CAD build for the part. Positions are in the model's coordinates, mm. A direction names the side the tool comes from. Give positions to 0.01 mm unless a question says otherwise; leave off trailing zeros. Loops run counter-clockwise (first coordinate to the right, second up) from the corner with the lowest first, then second, coordinate; pieces in that order, holes last.
Item 1: Saw through at A-A on x = -11. Give the cut face in (y, z), plus the area to 3 significant figures.
Item 2: Mould opens along X. For faces 1 (the flat face through (-11.5, 2, 0)), 2 (the flat face through (18.75, 2, 0)), 3 (the cylindrical face through (-17.32, 2.54, 7.5)), 4 (the flat face through (0, 0, 8)) say: released by +X, released by -X, zero draft, split by the parting line, or undercut.
Item 3: Saw through at B-B on y = 3.75. Give the cut face in (x, z).
Item 4: Saw through at D-D on z = 0.75. Give the cut face in (x, y).
Item 5: Probe probe 1 along X at (y, z) = (1.4, 0); probe 2 along Z at (x, y) = (2, 0.55); probe 3 along X at (y, z) = (2.9, -3). List the from-to ranges inside material, lowest first.
Item 6: Drop flat-ended pins along their axis: P1, Ø1, axis at y = 3, z = -6, coming from the -X side; P2, Ø3.5, axis at x = 14.1, z = 0, coming from the +Y side; P3, Ø3, axis at y = 1, z = -6.5, coming from the +X side. Give the stop position or say it passes through.
Item 7: Saw through at C-C on z = 4.5. Give the cut face in (x, y).
Item 8: Which spindle directions (+Z, -Z, +X, -X, +Y, -Y) get a long thin tool onto all of the face, cutting with end or side? Do faces 5 (the cylindrical face through (-16.85, 3.77, -0.06)), 6 (the flat face through (0, 2, 7.1)), 7 (the cylindrical face through (17.25, 2.54, 7.57)). Say none if no direction does.
from build123d import *

# Parameters (mm, degrees)
SKETCH1_W           = 37.5
SKETCH1_H           = 18
SKETCH1_R           = 1.55
SKETCH1_W_2         = 23
SKETCH1_H_2         = 14.2
BOSS_EXTRUDE1_DEPTH = 5
SKETCH2_R           = 1.55
CUT_EXTRUDE1_DEPTH  = 2.5
FILLET1_R           = 5


with BuildPart() as part:
    # Sketch1 → Boss-Extrude1 (new body)
    with BuildSketch(Plane(origin=(0, 0, 0), x_dir=(1, 0, 0), z_dir=(0, 1, 0))):
        Rectangle(SKETCH1_W, SKETCH1_H)
        with Locations((-14.1, 0)):
            Circle(SKETCH1_R, mode=Mode.SUBTRACT)
        with Locations((14.1, 0)):
            Circle(SKETCH1_R, mode=Mode.SUBTRACT)
        Rectangle(SKETCH1_W_2, SKETCH1_H_2, mode=Mode.SUBTRACT)
    extrude(amount=BOSS_EXTRUDE1_DEPTH)

    # Sketch2 → Cut-Extrude1 (cut)
    with BuildSketch(Plane(origin=(0, 5, 0), x_dir=(1, 0, 0), z_dir=(0, 1, 0))):
        with BuildLine():
            ThreePointArc((11.5, 0.895823643), (12.503286973, 2.238974656), (14.1, 2.75))
            Line((14.1, 2.75), (11.5, 2.75))
            Line((11.5, 2.75), (11.5, 0.895823643))
        make_face()
        with BuildLine():
            Line((11.5, -2.75), (14.1, -2.75))
            ThreePointArc((14.1, -2.75), (12.503286973, -2.238974656), (11.5, -0.895823643))
            Line((11.5, -0.895823643), (11.5, -2.75))
        make_face()
        with BuildLine():
            ThreePointArc((16.85, 0), (16.044543648, 1.944543648), (14.1, 2.75))
            ThreePointArc((14.1, 2.75), (12.503286973, 2.238974656), (11.5, 0.895823643))
            Line((11.5, 0.895823643), (11.5, -0.895823643))
            ThreePointArc((11.5, -0.895823643), (12.503286973, -2.238974656), (14.1, -2.75))
            ThreePointArc((14.1, -2.75), (16.044543648, -1.944543648), (16.85, 0))
        make_face()
        with Locations((14.1, 0)):
            Circle(SKETCH2_R, mode=Mode.SUBTRACT)
        with BuildLine():
            ThreePointArc((-11.5, -0.895823643), (-12.503286973, -2.238974656), (-14.1, -2.75))
            Line((-14.1, -2.75), (-11.5, -2.75))
            Line((-11.5, -2.75), (-11.5, -0.895823643))
        make_face()
        with BuildLine():
            Line((-11.5, 2.75), (-14.1, 2.75))
            ThreePointArc((-14.1, 2.75), (-12.503286973, 2.238974656), (-11.5, 0.895823643))
            Line((-11.5, 0.895823643), (-11.5, 2.75))
        make_face()
        with BuildLine():
            ThreePointArc((-11.5, 0.895823643), (-12.503286973, 2.238974656), (-14.1, 2.75))
            ThreePointArc((-14.1, 2.75), (-16.85, 0), (-14.1, -2.75))
            ThreePointArc((-14.1, -2.75), (-12.503286973, -2.238974656), (-11.5, -0.895823643))
            Line((-11.5, -0.895823643), (-11.5, 0.895823643))
        make_face()
        with Locations((-14.1, 0)):
            Circle(SKETCH2_R, mode=Mode.SUBTRACT)
    extrude(amount=-CUT_EXTRUDE1_DEPTH, mode=Mode.SUBTRACT)

    # Fillet1
    fillet1_edges = [part.edges().sort_by_distance(p)[0] for p in [
        (18.75, 2.5, 9),
        (-18.75, 2.5, 9),
        (-18.75, 2.5, -9),
        (18.75, 2.5, -9),
    ]]
    fillet(fillet1_edges, radius=FILLET1_R)


solid = part.part
Results below:
1. outline: (0, -9) - (5, -9) - (5, -7.1) - (0, -7.1) - close; (0, 7.1) - (5, 7.1) - (5, 9) - (0, 9) - close
1. area: 19.0 mm2
2. face 1: undercut
2. face 2: released by +X
2. face 3: released by -X
2. face 4: zero draft
3. outline: (-18.75, -4) arc R5 ccw to (-13.75, -9) - (13.75, -9) arc R5 ccw to (18.75, -4) - (18.75, 4) arc R5 ccw to (13.75, 9) - (-13.75, 9) arc R5 ccw to (-18.75, 4) - close; hole (-14.1, -2.75) - (-11.5, -2.75) - (-11.5, -7.1) - (11.5, -7.1) - (11.5, -2.75) - (14.1, -2.75) arc R2.75 ccw to (14.1, 2.75) - (11.5, 2.75) - (11.5, 7.1) - (-11.5, 7.1) - (-11.5, 2.75) - (-14.1, 2.75) arc R2.75 ccw to start
4. outline: (-18.75, 0) - (-15.46, 0) - (-15.46, 2.5) - (-16.75, 2.5) - (-16.75, 5) - (-18.75, 5) - close; (-12.74, 0) - (-11.5, 0) - (-11.5, 2.5) - (-12.74, 2.5) - close; (11.5, 0) - (12.74, 0) - (12.74, 2.5) - (11.5, 2.5) - close; (15.46, 0) - (18.75, 0) - (18.75, 5) - (16.75, 5) - (16.75, 2.5) - (15.46, 2.5) - close
5. probe 1: x = -18.75 to -15.65, -12.55 to -11.5, 11.5 to 12.55, 15.65 to 18.75
5. probe 2: z = -9 to -7.1, 7.1 to 9
5. probe 3: x = -18.75 to -11.5, 11.5 to 18.75
6. P1: stops at x = -18.52
6. P2: stops at y = 2.5
6. P3: stops at x = 18.65
7. outline: (-18.72, 0) - (-11.5, 0) - (-11.5, 5) - (-18.72, 5) - close; (11.5, 0) - (18.72, 0) - (18.72, 5) - (11.5, 5) - close
8. face 5: +Y
8. face 6: +Y, -Y
8. face 7: +Z, +X, +Y, -Y
